from build123d import *

# Parameters (mm, degrees)
SKETCH1_W           = 18
SKETCH1_H           = 5
BOSS_EXTRUDE1_DEPTH = 3.4
SKETCH2_W           = 27.5
SKETCH2_H           = 4
BOSS_EXTRUDE2_DEPTH = 8.7
SKETCH3_W           = 2
SKETCH3_H           = 8.7
BOSS_EXTRUDE3_DEPTH = 23.8
SKETCH4_W           = 27.5
SKETCH4_H           = 8.7
BOSS_EXTRUDE4_DEPTH = 5
SKETCH5_R           = 1.05
SKETCH5_R_2         = 1
CUT_EXTRUDE1_DEPTH  = 39.869557497


with BuildPart() as part:
    # Sketch1 → Boss-Extrude1 (new body)
    with BuildSketch(Plane.XY):
        Rectangle(SKETCH1_W, SKETCH1_H)
    extrude(amount=BOSS_EXTRUDE1_DEPTH)

    # Sketch2 → Boss-Extrude2 (add)
    with BuildSketch(Plane.XY.offset(3.4)):
        with Locations((0, 4.5)):
            Rectangle(SKETCH2_W, SKETCH2_H)
    extrude(amount=-BOSS_EXTRUDE2_DEPTH)

    # Sketch3 → Boss-Extrude3 (add)
    with BuildSketch(Plane(origin=(0, 6.5, 0), x_dir=(1, 0, 0), z_dir=(0, 1, 0))):
        with Locations((-12.75, 0.95)):
            Rectangle(SKETCH3_W, SKETCH3_H)
        with Locations((12.75, 0.95)):
            Rectangle(SKETCH3_W, SKETCH3_H)
    extrude(amount=BOSS_EXTRUDE3_DEPTH)

    # Sketch4 → Boss-Extrude4 (add)
    with BuildSketch(Plane(origin=(0, 30.3, 0), x_dir=(1, 0, 0), z_dir=(0, 1, 0))):
        with Locations((0, 0.95)):
            Rectangle(SKETCH4_W, SKETCH4_H)
    extrude(amount=BOSS_EXTRUDE4_DEPTH)

    # Sketch5 → Cut-Extrude1 (cut, through all)
    with BuildSketch(Plane.XY.offset(3.4)):
        with Locations((-4.5, -0.5)):
            Circle(SKETCH5_R)
        with Locations((4.5, -0.5)):
            Circle(SKETCH5_R)
        with Locations((-6, 4.5)):
            Circle(SKETCH5_R_2)
        with Locations((6, 4.5)):
            Circle(SKETCH5_R_2)
        with Locations(Location((6, 32.3, 0), (0, 0, 180))):
            Circle(SKETCH5_R_2)
        with Locations(Location((-6, 32.3, 0), (0, 0, 180))):
            Circle(SKETCH5_R_2)
    extrude(amount=-CUT_EXTRUDE1_DEPTH, mode=Mode.SUBTRACT)


solid = part.part
Input: part model. Units: mm. Frame: model coordinates. A direction names the side the tool comes from. Give positions to 0.01 mm unless a question says otherwise; leave off trailing zeros. Loops run counter-clockwise (first coordinate to the right, second up) from the corner with the lowest first, then second, coordinate; pieces in that order, holes last. Notation, with made-up numbers: M 77.25,-0.75 L 106.25,-0.75 A23 ccw 106.25,35.25 Z; hole C 27.5,8.25 d10. An arc over 180 degrees is marked long. Use one line per item in the form item = value.
1. Section query C-C, the plane y = 19.5. Return the cut outline in (x, z).
Numbers:
outline = M -13.75,-5.3 L -11.75,-5.3 L -11.75,3.4 L -13.75,3.4 Z; M 11.75,-5.3 L 13.75,-5.3 L 13.75,3.4 L 11.75,3.4 Z
2. Section query A-A, the plane x = 4.5. Return the cut outline in (y, z).
Numbers:
outline = M -2.5,0 L -1.55,0 L -1.55,3.4 L -2.5,3.4 Z; M 0.55,0 L 2.5,0 L 2.5,-5.3 L 6.5,-5.3 L 6.5,3.4 L 0.55,3.4 Z; M 30.3,-5.3 L 35.3,-5.3 L 35.3,3.4 L 30.3,3.4 Z
3. Pull-direction query (Y, two-part tool) for faces 1 (the face through (0, -2.5, 2)), 2 (the face through (-6.737, 5.176, -0.889)), 3 (the face through (-1, 31, -5.3)); classes: released by +Y, released by -Y, zero draft, split by the parting line, or undercut.
Numbers:
face_1 = released by -Y
face_2 = undercut
face_3 = zero draft
4. Line query: L1, parallel to X at y = 32.3, z = 0.5; L2, parallel to Y at x = -6, z = 0.5; L3, parallel to Y at x = -6, z = -1. Output: solid intervals per line, ascending.
Numbers:
L1 = -13.75 to -7, -5 to 5, 7 to 13.75
L2 = -2.5 to 3.5, 5.5 to 6.5, 30.3 to 31.3, 33.3 to 35.3
L3 = 2.5 to 3.5, 5.5 to 6.5, 30.3 to 31.3, 33.3 to 35.3
5. Section query D-D, the plane x = 8.25. Return the cut outline in (y, z).
Numbers:
outline = M -2.5,0 L 2.5,0 L 2.5,-5.3 L 6.5,-5.3 L 6.5,3.4 L -2.5,3.4 Z; M 30.3,-5.3 L 35.3,-5.3 L 35.3,3.4 L 30.3,3.4 Z
6. Reachability of faces 4 (the face through (9, 0, 2)), 5 (the face through (13.75, 19, -1)), 6 (the face through (0, 0, 0)), 7 (the face through (0, 6.5, -1)), 8 (the face through (-9, 0, 2)) from +Z, -Z, +X, -X, +Y, -Y: full face, straight path, thin tool, end or side. Return the list, or none.
Numbers:
face_4 = +Z, -Z, +X, -Y
face_5 = +Z, -Z, +X, +Y, -Y
face_6 = -Z, +X, -X, -Y
face_7 = +Z, -Z
face_8 = +Z, -Z, -X, -Y
7. First-contact query: pin 1 (2.5 mm diameter, centred on x = -4.5, y = -0.5, fed in from -Z); pin 2 (1.7 mm diameter, centred on y = -0.5, z = 1.5, fed in from +X); pin 3 (1 mm diameter, centred on y = 0, z = 1.5, fed in from -X); pin 4 (1.9 mm diameter, centred on x = 4.5, y = -0.5, fed in from -Z). Flat tips, straight axial feed; report the tip coordinate or a pass-through.
Numbers:
pin_1 = 0
pin_2 = 9
pin_3 = -9
pin_4 = through
8. Section query B-B, the plane z = -4.5. Return the cut outline in (x, y).
Numbers:
outline = M -13.75,2.5 L 13.75,2.5 L 13.75,35.3 L -13.75,35.3 Z; hole M -11.75,6.5 L 11.75,6.5 L 11.75,30.3 L -11.75,30.3 Z; hole C -6,4.5 d2; hole C -6,32.3 d2; hole C 6,4.5 d2; hole C 6,32.3 d2
